from build123d import *

# Parameters (mm, degrees)
F0_W     = 1270
F0_H     = 381
F1_DEPTH = 25.4
F2_W     = 25.4
F2_H     = 6.35
F3_DEPTH = 25.4
F4_R     = 12.69999
F5_R     = 3.175
F6_DEPTH = 381.001


# Not quite as in the source:
# - a fillet or chamfer is up to 0.001 mm smaller than in the source, because OpenCascade refuses the exact size


with BuildPart() as f1:
    # F0 (on Top) → F1 (new body)
    with BuildSketch(Plane.XY):
        Rectangle(F0_W, F0_H)
    extrude(amount=F1_DEPTH)

    # F2 (on face) → F3 (join)
    with BuildSketch(Plane(origin=(0, 0, 0), x_dir=(1, 0, 0), z_dir=(0, 0, -1))):
        with Locations((-406.4, 187.325)):
            Rectangle(F2_W, F2_H)
        with Locations((-406.4, -187.325)):
            Rectangle(F2_W, F2_H)
    extrude(amount=F3_DEPTH)

    # F4 (radius 12.7 in the source; OpenCascade refuses exactly that, so slightly less here)
    f4_edges = [f1.edges().sort_by_distance(p)[0] for p in [
        (-419.1, -187.325, -25.4),
        (-393.7, -187.325, -25.4),
        (-419.1, 187.325, -25.4),
        (-393.7, 187.325, -25.4),
    ]]
    fillet(f4_edges, radius=F4_R)

    # F5 (on face) → F6 (cut, through all)
    with BuildSketch(Plane(origin=(0, 190.5, 0), x_dir=(-1, 0, 0), z_dir=(0, 1, 0))):
        with Locations((406.4, -12.7)):
            Circle(F5_R)
    extrude(amount=-F6_DEPTH, mode=Mode.SUBTRACT)


solid = f1.part
Check sheet for the modelled part. Datum: model origin and axes. Units: mm. A direction names the side the tool comes from. Give positions to 0.01 mm unless a question says otherwise; leave off trailing zeros. Write each loop counter-clockwise with the first axis right and the second up, starting at its lowest first coordinate (ties: lowest second). Pieces come first, ordered by that corner, then holes. Notation, with made-up numbers: (-10, 57.5) -> (27, 57.5) arc R15 ccw to (27, 84.5) -> close; hole circle Ø8 at (14, 35). An arc over 180 degrees is marked (long way). One line per item, written item: value. Start each with the question number.
Item 1: Section check B-B on x = -110. Record the cut outline in (y, z), then the cut area to 3 significant figures.
Item 2: Section check A-A on y = -95. Record the cut outline in (x, z).
Item 3: Draft check along Y on faces 3 (the flat face through (-9, 190.5, 17)), 4 (the flat face through (-635, -3, 13)), 5 (the flat face through (-9, -190.5, 17)), 6 (the flat face through (-404, 184.15, -10)). Enter one of: +Y half, -Y half, draft (parallel to the pull), parting line (faces both ways), or undercut.
Item 4: Gauge pin test, flat ends, axial feed: pin 1 (7 mm diameter, centred on y = -186, z = -4.5, fed in from -X); pin 2 (1.9 mm diameter, centred on y = -188.5, z = -5.5, fed in from +X); pin 3 (10 mm diameter, centred on x = -406.4, z = -12.7, fed in from -Y). Record the tip position at first contact, or that the pin passes through.
Item 5: Tool access check on faces 1 (the flat face through (-404, -184.15, -10)), 2 (the flat face through (-9, 3, 25.4)). Record the directions out of +Z, -Z, +X, -X, +Y, -Y that give a thin tool (end or side, any length) a straight path to the whole face; none if there is none.
Item 6: Material ranges on probe 1 along X at (y, z) = (187, -12); probe 2 along Y at (x, z) = (-395.5, -7.5); probe 3 along Z at (x, y) = (-1, 35), recorded low to high. Write a range as from..to.
Results list:
1. outline: (-190.5, 0) -> (190.5, 0) -> (190.5, 25.4) -> (-190.5, 25.4) -> close
1. area: 9,680 mm²
2. outline: (-635, 0) -> (635, 0) -> (635, 25.4) -> (-635, 25.4) -> close
3. face 3: +Y half
3. face 4: draft
3. face 5: -Y half
3. face 6: undercut
4. pin 1: x = -419.1
4. pin 2: x = -393.7
4. pin 3: y = -190.5
5. face 1: -Z, +X, -X
5. face 2: +Z, +X, -X, +Y, -Y
6. probe 1: -419.1..-409.5, -403.3..-393.7
6. probe 2: -190.5..-184.15, 184.15..190.5
6. probe 3: 0..25.4
